Geometry: final body of the model. Coordinates: model frame, mm. Face numbers are marked on the shaded views. A direction names the side the tool comes from. Give positions to 0.01 mm unless a question says otherwise; leave off trailing zeros. Loops run counter-clockwise (first coordinate to the right, second up) from the corner with the lowest first, then second, coordinate; pieces in that order, holes last. Notation, with made-up numbers: (79.5, 70) - (85.5, 70) arc R22 ccw to (85.5, 91) - close; hole circle Ø5 at (56.25, -22). An arc over 180 degrees is marked (long way). Answer in a Markdown table with one row per item.
from build123d import *

# Parameters (mm, degrees)
VACIADO1_T = -10


with BuildPart() as part:
    # Croquis1 → Revolución1 (revolve)
    with BuildSketch(Plane.XY, mode=Mode.PRIVATE) as revoluci_n1_sk:
        Polygon((0, 53.427911052), (0, -72.710427761), (17.703234608, -72.710427761), (17.703234608, -9.641258354), (52.203454236, 24.858961274), (52.203454236, 53.427911052), align=None)
    revolve(revoluci_n1_sk.sketch.rotate(Axis((52.203454236, 53.427911052, 0), (-1, 0, 0)), 270), axis=Axis((52.203454236, 53.427911052, 0), (-1, 0, 0)))

    # Vaciado1
    vaciado1_openings = [part.faces().sort_by_distance(p)[0] for p in [
        (52.203454236, 53.427911052, 0),
        (0, 53.427911052, 0),
    ]]
    offset(amount=VACIADO1_T, openings=vaciado1_openings, kind=Kind.INTERSECTION)


solid = part.part
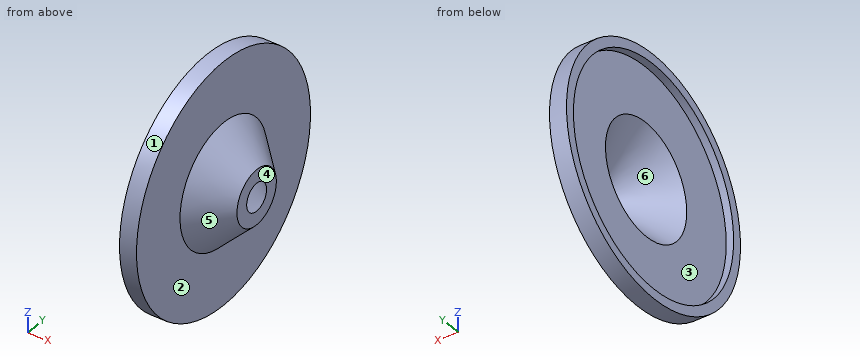
Q1. Cut plane A-A (z = 0). Output: boundary loops of the cut face in (x, y).
Check values:
| item | result |
|---|---|
| outline | (0, -72.71) - (17.7, -72.71) - (17.7, -9.64) - (52.2, 24.86) - (52.2, 39) - (7.7, -5.5) - (7.7, -62.71) - (0, -62.71) - close; (0, 169.57) - (7.7, 169.57) - (7.7, 112.35) - (52.2, 67.85) - (52.2, 82) - (17.7, 116.5) - (17.7, 179.57) - (0, 179.57) - close |
Q2. Reachability of the marked faces 1, 2 and 3 from +Z, -Z, +X, -X, +Y, -Y: full face, straight path, thin tool, end or side. Return the list, or none.
Check values:
| item | result |
|---|---|
| face 1 | +X, -X |
| face 2 | +X |
| face 3 | -X |
Q3. First-contact query: pin 1 (3 mm diameter, centred on y = 38.5, z = -18, fed in from -X); pin 2 (12 mm diameter, centred on x = 14.5, y = -43.5, fed in from +Z); pin 3 (2 mm diameter, centred on y = -17.5, z = 42.5, fed in from +X); pin 4 (2 mm diameter, centred on y = 38, z = -25, fed in from +X). Flat tips, straight axial feed; report the tip coordinate or a pass-through.
Check values:
| item | result |
|---|---|
| pin 1 | x = 41.75 |
| pin 2 | z = 87.42 |
| pin 3 | x = 17.7 |
| pin 4 | x = 52.2 |
Q4. Cut plane D-D (x = 42.5). Output: boundary loops of the cut face in (y, z), and give its area (3 significant figures).
Check values:
| item | result |
|---|---|
| outline | circle Ø76.54 at (53.43, 0); hole circle Ø48.26 at (53.43, 0) |
| area | 2,770 mm² |
Q5. Material intervals for line 1 along Y through (x, z) = (2, 0); line 2 along X through (y, z) = (150, -49); line 3 along Z through (x, y) = (22.5, 43.5), sorted ascending.
Check values:
| item | result |
|---|---|
| line 1 | -72.71 to -62.71, 169.57 to 179.57 |
| line 2 | 7.7 to 17.7 |
| line 3 | -57.42 to -43, 43 to 57.42 |
Q6. Cut plane B-B (y = 128). Output: boundary loops of the cut face in (x, z).
Check values:
| item | result |
|---|---|
| outline | (0, -101.73) - (17.7, -101.73) - (17.7, 101.73) - (0, 101.73) - (0, 89.03) - (7.7, 89.03) - (7.7, -89.03) - (0, -89.03) - close |
Q7. Draft query along Z for the marked faces 4, 5 and 6. Return one class per face: pulls with the +Z half, pulls with the -Z half, needs draft (parallel to the pull), parting line crosses it, or undercut.
Check values:
| item | result |
|---|---|
| face 4 | needs draft |
| face 5 | parting line crosses it |
| face 6 | undercut |
Q8. Cut plane C-C (z = -68.5). Output: boundary loops of the cut face in (x, y).
Check values:
| item | result |
|---|---|
| outline | (0, -52.49) - (17.7, -52.49) - (17.7, 159.35) - (0, 159.35) - (0, 147.21) - (7.7, 147.21) - (7.7, -40.36) - (0, -40.36) - close |
